from build123d import *

# Parameters (mm, degrees)
SKETCH_W            = 43
SKETCH_H            = 43
PAD_DEPTH           = 20
HOLE_D              = 3.75
HOLE_CBORE_D        = 5.75
HOLE_CBORE_DEPTH    = 15
HOLE001_D           = 25
HOLE001_CSINK_D     = 30
HOLE001_CSINK_ANGLE = 90
SKETCH003_W         = 20
SKETCH003_H         = 32.696217
POCKET_DEPTH        = 5
POCKET001_DEPTH     = 25
SKETCH005_W         = 11.5
SKETCH005_H         = 11.5
PAD001_DEPTH        = 10
PAD001_DEPTH_BACK   = 2
HOLE002_D           = 3.75
HOLE002_CBORE_D     = 5.75
HOLE002_CBORE_DEPTH = 15
SKETCH007_R         = 2.75
HOLE003_DEPTH       = 11.501
POCKET002_DEPTH     = 2.5


with BuildPart() as part:
    # Sketch → Pad (new body)
    with BuildSketch(Plane.XY):
        with Locations((21.5, 21.5)):
            Rectangle(SKETCH_W, SKETCH_H)
    extrude(amount=PAD_DEPTH)

    # Hole (through all)
    with Locations(Plane.XY.offset(20)):
        with Locations((6, 37), (37, 37), (37, 6), (6, 6)):
            CounterBoreHole(HOLE_D / 2, HOLE_CBORE_D / 2, HOLE_CBORE_DEPTH)

    # Hole001 (through all)
    with Locations(Plane.XY.offset(20)):
        with Locations((21.5, 21.5)):
            CounterSinkHole(HOLE001_D / 2, HOLE001_CSINK_D / 2, counter_sink_angle=HOLE001_CSINK_ANGLE)

    # Sketch003 (on Face5 of Hole001) → Pocket (cut)
    with BuildSketch(Plane.XY.offset(20)):
        with Locations((21.5, 34.162118)):
            Rectangle(SKETCH003_W, SKETCH003_H)
    extrude(amount=-POCKET_DEPTH, mode=Mode.SUBTRACT)

    # Sketch004 (on Face1 of Pocket) → Pocket001 (cut)
    with BuildSketch(Plane.XZ):
        with BuildLine():
            ThreePointArc((16.5, 14), (21.5, 9), (26.5, 14))
            Line((26.5, 20), (26.5, 14))
            Line((16.5, 20), (26.5, 20))
            Line((16.5, 20), (16.5, 14))
        make_face()
    extrude(amount=-POCKET001_DEPTH, mode=Mode.SUBTRACT)

    # Sketch005 (on Face8 of Pocket001) → Pad001 (join, two sides)
    with BuildSketch(Plane.XY.offset(20)) as pad001_sk:
        with Locations((5.75, 37.25)):
            Rectangle(SKETCH005_W, SKETCH005_H)
        with Locations((37.25, 37.25)):
            Rectangle(SKETCH005_W, SKETCH005_H)
    extrude(amount=PAD001_DEPTH)
    extrude(pad001_sk.sketch, amount=-PAD001_DEPTH_BACK)

    # Hole002 (through all)
    with Locations(Plane.XY.offset(30)):
        with Locations((6, 37), (37, 37)):
            CounterBoreHole(HOLE002_D / 2, HOLE002_CBORE_D / 2, HOLE002_CBORE_DEPTH)

    # Sketch007 (on Face22 of Hole002) → Hole003 (cut, through all)
    with BuildSketch(Plane.XZ.offset(-31.5)):
        with Locations((5.75, 25)):
            Circle(SKETCH007_R)
        with Locations((37.25, 25)):
            Circle(SKETCH007_R)
    extrude(amount=-HOLE003_DEPTH, mode=Mode.SUBTRACT)

    # Sketch008 → Pocket002 (cut, symmetric)
    with BuildSketch(Plane.YZ.offset(30.5)):
        with BuildLine():
            Line((7, 20), (7, 19))
            ThreePointArc((1, 13), (5.242641, 14.757359), (7, 19))
            Line((1, 13), (0, 13))
            Line((0, 16), (0, 13))
            Line((1, 16), (0, 16))
            ThreePointArc((1, 16), (3.12132, 16.87868), (4, 19))
            Line((4, 20), (4, 19))
            Line((4, 20), (7, 20))
        make_face()
    extrude(amount=POCKET002_DEPTH, both=True, mode=Mode.SUBTRACT)


solid = part.part
Input: part model. Units: mm. Frame: model coordinates. A direction names the side the tool comes from. Coordinates: 2 decimals unless noted, no trailing zeros. Loops run counter-clockwise (first coordinate to the right, second up) from the corner with the lowest first, then second, coordinate; pieces in that order, holes last. Notation, with made-up numbers: (-4.5, 59.25) - (7.5, 59.25) arc R25 ccw to (7.5, 96.25) - close; hole circle Ø3 at (52, 3.25). An arc over 180 degrees is marked (long way). Answer in a Markdown table with one row per item. Add a question column.
Item 1: Contact query for flat-ended pins moving along their axis: P1, Ø1.7, axis at x = 4.5, y = 5.5, coming from the +Z side; P2, Ø6.5, axis at x = 6, y = 37, coming from the +Z side; P3, Ø2, axis at x = 14, z = 22.5, coming from the +Y side; P4, Ø12, axis at x = 11.5, y = 10.5, coming from the +Z side. Output: stop coordinate, or through.
Item 2: Section query B-B on y = 21.5. Return the cut outline in (x, z), then the cut area to 3 significant figures.
Item 3: Line query: line 1 along Y through (x, z) = (37, 17.25) (3 decimals); line 2 along Y through (x, z) = (37, 1.45) (3 decimals); line 3 along X through (y, z) = (21.5, 4.5). Output: solid intervals per line, ascending. Write a range as [from, to].
Item 4: Section query A-A on x = 21.5. Return the cut outline in (y, z), then the cut area to 3 significant figures.
Item 5: Access query for faces 5 (the flat face through (31, 12, 0)), 6 (the cylindrical face through (30.535, 5.196, 14.711)), 7 (the flat face through (8, 36, 5)), 8 (the flat face through (6, 12, 20)), 9 (the flat face through (11.5, 37, 22)). Directions: +Z, -Z, +X, -X, +Y, -Y. A direction counts if a zero-diameter tool reaches every point of the face in a straight line with its end or side. Return the directions, or none.
Item 6: Mould query, pull axis Y, two halves, no side actions, for faces 1 (the flat face through (21, 43, 12)), 2 (the cylindrical face through (30.54, 3.1, 16.86)), 3 (the flat face through (21, 0, 8)), 4 (the flat face through (21, 38, 15)). Classes: released by +Y, released by -Y, zero draft, split by the parting line, or undercut.
Item 7: Section query C-C on z = 2. Return the cut outline in (x, y) (3 decimals), then the cut area to 3 significant figures.
Item 8: Section query D-D on x = 37.25. State how many separate pieces and enclosed holes the cut face has, then the cut area to 3 significant figures.
Recorded:
| question | item | result |
|---|---|---|
| 1 | P1 | z = 5 |
| 1 | P2 | z = 30 |
| 1 | P3 | through |
| 1 | P4 | z = 20 |
| 2 | outline | (0, 0) - (9, 0) - (9, 17.5) - (6.5, 20) - (0, 20) - close; (34, 0) - (43, 0) - (43, 20) - (36.5, 20) - (34, 17.5) - close |
| 2 | area | 354 mm^2 |
| 3 | line 1 | [0, 3.125], [8.875, 34.125], [39.875, 43] |
| 3 | line 2 | [0, 4.125], [7.875, 35.125], [38.875, 43] |
| 3 | line 3 | [0, 9], [34, 43] |
| 4 | outline | (0, 0) - (9, 0) - (9, 9) - (0, 9) - close; (34, 0) - (43, 0) - (43, 15) - (34, 15) - close |
| 4 | area | 216 mm^2 |
| 5 | face 5 | -Z, +X, -X, +Y, -Y |
| 5 | face 6 | none |
| 5 | face 7 | +Z |
| 5 | face 8 | +Z, +X, -X, -Y |
| 5 | face 9 | +Z, +Y |
| 6 | face 1 | released by +Y |
| 6 | face 2 | undercut |
| 6 | face 3 | released by -Y |
| 6 | face 4 | zero draft |
| 7 | outline | (0, 0) - (43, 0) - (43, 43) - (0, 43) - close; hole circle Ø3.75 at (6, 6); hole circle Ø3.75 at (6, 37); hole circle Ø25 at (21.5, 21.5); hole circle Ø3.75 at (37, 6); hole circle Ø3.75 at (37, 37) |
| 7 | area | 1,310 mm^2 |
| 8 | separate pieces | 5 |
| 8 | enclosed holes | 0 |
| 8 | area | 677 mm^2 |
